```python
from build123d import *

# Parameters (mm, degrees)
SKETCH1_R           = 13.5
SKETCH1_R_2         = 4
BOSS_EXTRUDE1_DEPTH = 4
CUT_EXTRUDE1_DEPTH  = 20.506409203
CIRPATTERN1_COUNT   = 5
CHAMFER1_SIZE       = 0.5
SKETCH4_R           = 13.5
SKETCH4_R_2         = 13.2
CUT_EXTRUDE3_DEPTH  = 2.5
CHAMFER2_SIZE       = 0.5
CHAMFER2_SIZE2      = 1.5


with BuildPart() as part:
    # Sketch1 → Boss-Extrude1 (new, symmetric)
    with BuildSketch(Plane(origin=(0, 0, 0), x_dir=(0, 0, -1), z_dir=(1, 0, 0))):
        Circle(SKETCH1_R)
        Circle(SKETCH1_R_2, mode=Mode.SUBTRACT)
    extrude(amount=BOSS_EXTRUDE1_DEPTH, both=True)

    # Sketch2 → Cut-Extrude1 (cut, symmetric)
    with BuildSketch(Plane(origin=(0, 0, 0), x_dir=(0, 0, -1), z_dir=(1, 0, 0))):
        with BuildLine():
            ThreePointArc((0, 5.849695328), (-2.956289657, 7.377375059), (-5.012219469, 9.99397715))
            ThreePointArc((-5.012219469, 9.99397715), (-2.621563936, 11.159720287), (0, 11.6087119))
            ThreePointArc((0, 11.6087119), (2.621563936, 11.159720287), (5.012219469, 9.99397715))
            ThreePointArc((5.012219469, 9.99397715), (2.956289657, 7.377375059), (0, 5.849695328))
        make_face()
    cut_extrude1 = extrude(amount=CUT_EXTRUDE1_DEPTH, both=True, mode=Mode.SUBTRACT)

    # CirPattern1: Cut-Extrude1 ×5 about axis
    cirpattern1_axis = Axis((0, 0, 0), (1, 0, 0))
    for i in range(1, CIRPATTERN1_COUNT):
        add(cut_extrude1.rotate(cirpattern1_axis, i * 360 / CIRPATTERN1_COUNT), mode=Mode.SUBTRACT)

    # Chamfer1
    chamfer1_edges = [part.edges().sort_by_distance(p)[0] for p in [
        (4, 0, 13.5),
    ]]
    chamfer(chamfer1_edges, length=CHAMFER1_SIZE)

    # Sketch4 → Cut-Extrude3 (cut, symmetric)
    with BuildSketch(Plane(origin=(0, 0, 0), x_dir=(0, 0, -1), z_dir=(1, 0, 0))):
        Circle(SKETCH4_R)
        Circle(SKETCH4_R_2, mode=Mode.SUBTRACT)
    extrude(amount=CUT_EXTRUDE3_DEPTH, both=True, mode=Mode.SUBTRACT)

    # Chamfer2
    chamfer2_edges = [part.edges().sort_by_distance(p)[0] for p in [
        (4, 0, 4),
    ]]
    chamfer2_side = [part.faces().sort_by_distance(p)[0] for p in [
        (4, 0, 12.632304474),
    ]]
    chamfer(chamfer2_edges, length=CHAMFER2_SIZE, length2=CHAMFER2_SIZE2, reference=chamfer2_side[0])


solid = part.part
```
Can you work these out from the model? Positions are in its coordinate system, mm. Coordinates: 2 decimals unless noted, no trailing zeros. Loops run counter-clockwise (first coordinate to the right, second up) from the corner with the lowest first, then second, coordinate; pieces in that order, holes last. Notation, with made-up numbers: (47.5, 8.5) -> (93.5, 8.5) arc R28 cw to (93.5, 45.5) -> close; hole circle Ø4 at (63, -13). An arc over 180 degrees is marked (long way). Put each result on its own line as item: value. Start each with the question number.
Q1. I want a section at C-C (x = -3.5). Write out the boundary of the cut face in (y, z).
Q2. If I drill on line 1 (Y direction, x = 0.5, z = -6.75); line 2 (Z direction, x = -3.5, y = -6.75); line 3 (Y direction, x = 2.25, z = 6.5), over which ranges is the centre line in solid material (lowest first)? Write a range as [from, to].
Q3. I want a section at D-D (y = -8). Count the separate pieces of the cut face and the enclosed holes in it, plus the area to 3 significant figures.
Q4. I'm going to push flat-ended pins straight in: P1, Ø3, axis at x = -2, y = -7.5, coming from the -Z side; P2, Ø1.5, axis at y = 1.5, z = 2, coming from the +X side. Where does each tip first touch, or does it pass through?
Q5. I want a section at A-A (x = -0.75). Write out the boundary of the cut face in (y, z).
Q6. I want a section at B-B (y = 0). Write out the boundary of the cut face in (x, z), plus the area to 3 significant figures.
Q7. Thinking about a two-plate mould opening in X: for faces 1 (the face through (0.056, 11.148, 2.657)), 2 (the face through (-0.04, 8.92, 9.73)), 3 (the face through (-4, 3, -3)), 4 (the face through (4, 0, -6)), which applies, pulls with the +X half, pulls with the -X half, needs draft (parallel to the pull), parting line crosses it, or undercut?
Taken from the geometry:
1. outline: circle Ø27 at (0, 0); hole (-11.03, -1.82) arc R9.39 ccw to (-9.39, -6.82) arc R9.39 ccw to (-5.14, -9.93) arc R7.84 ccw to (-4.73, -3.44) arc R7.84 ccw to start; hole (-11.03, 1.82) arc R7.84 ccw to (-4.73, 3.44) arc R7.84 ccw to (-5.14, 9.93) arc R9.39 ccw to (-9.39, 6.82) arc R9.39 ccw to start; hole circle Ø8 at (0, 0); hole (-1.68, -11.05) arc R9.39 ccw to (3.59, -11.04) arc R9.39 ccw to (7.86, -7.96) arc R7.84 ccw to (1.81, -5.56) arc R7.84 ccw to start; hole (-1.68, 11.05) arc R7.84 ccw to (1.81, 5.56) arc R7.84 ccw to (7.86, 7.96) arc R9.39 ccw to (3.59, 11.04) arc R9.39 ccw to start; hole (5.85, 0) arc R7.84 ccw to (9.99, -5.01) arc R9.39 ccw to (11.61, 0) arc R9.39 ccw to (9.99, 5.01) arc R7.84 ccw to start
2. line 1: y = [-11.34, -9.44], [-4.23, 0.39], [6.37, 11.34]
2. line 2: z = [-11.69, -9.17], [-2.26, 2.26], [9.17, 11.69]
2. line 3: y = [-11.49, -9.6], [-4.22, 0.63], [5.94, 11.49]
3. separate pieces: 3
3. enclosed holes: 0
3. area: 67.5 mm2
4. P1: stops at z = -12.05
4. P2: passes through
5. outline: circle Ø26.4 at (0, 0); hole (-11.03, -1.82) arc R9.39 ccw to (-9.39, -6.82) arc R9.39 ccw to (-5.14, -9.93) arc R7.84 ccw to (-4.73, -3.44) arc R7.84 ccw to start; hole (-11.03, 1.82) arc R7.84 ccw to (-4.73, 3.44) arc R7.84 ccw to (-5.14, 9.93) arc R9.39 ccw to (-9.39, 6.82) arc R9.39 ccw to start; hole circle Ø8 at (0, 0); hole (-1.68, -11.05) arc R9.39 ccw to (3.59, -11.04) arc R9.39 ccw to (7.86, -7.96) arc R7.84 ccw to (1.81, -5.56) arc R7.84 ccw to start; hole (-1.68, 11.05) arc R7.84 ccw to (1.81, 5.56) arc R7.84 ccw to (7.86, 7.96) arc R9.39 ccw to (3.59, 11.04) arc R9.39 ccw to start; hole (5.85, 0) arc R7.84 ccw to (9.99, -5.01) arc R9.39 ccw to (11.61, 0) arc R9.39 ccw to (9.99, 5.01) arc R7.84 ccw to start
6. outline: (-4, -13.5) -> (-2.5, -13.5) -> (-2.5, -13.2) -> (2.5, -13.2) -> (2.5, -13.5) -> (3.5, -13.5) -> (4, -13) -> (4, -11.38) -> (-4, -11.38) -> close; (-4, -7.19) -> (4, -7.19) -> (4, -4.5) -> (2.5, -4) -> (-4, -4) -> close; (-4, 4) -> (2.5, 4) -> (4, 4.5) -> (4, 7.19) -> (-4, 7.19) -> close; (-4, 11.38) -> (4, 11.38) -> (4, 13) -> (3.5, 13.5) -> (2.5, 13.5) -> (2.5, 13.2) -> (-2.5, 13.2) -> (-2.5, 13.5) -> (-4, 13.5) -> close
6. area: 81.0 mm2
7. face 1: needs draft
7. face 2: undercut
7. face 3: pulls with the -X half
7. face 4: pulls with the +X half
